```python
from build123d import *

# Parameters (mm, degrees)
F0_R     = 16.327253737
F0_R_2   = 12.7
F1_DEPTH = 101.6
F2_R     = 16.327253737
F3_DEPTH = 38.1
F3_TAPER = 22
F4_W     = 6.20650989
F4_H     = 11.6034736857
F5_DEPTH = 25.4
F7_DEPTH = 12.7
F8_COUNT = 3
F8_ANGLE = 240


with BuildPart() as f1:
    # F0 (on Front) → F1 (new body)
    with BuildSketch(Plane.XZ):
        Circle(F0_R)
        Circle(F0_R_2, mode=Mode.SUBTRACT)
    extrude(amount=F1_DEPTH)

    # F2 (on face) → F3 (join)
    with BuildSketch(Plane.XZ.offset(101.6)):
        Circle(F2_R)
    extrude(amount=F3_DEPTH, taper=F3_TAPER)

    # F4 (on Front) → F5 (join)
    with BuildSketch(Plane.XZ):
        with Locations((0.1349233789, 19.4290732034)):
            Rectangle(F4_W, F4_H)
    extrude(amount=F5_DEPTH)

    # F6 (on Right) → F7 (cut, symmetric)
    with BuildSketch(Plane.YZ):
        Polygon((25.9975232184, 33.8659547269), (-25.5434866995, 34.4056524336), (-25.8133374155, 16.5956672281), align=None)
    extrude(amount=F7_DEPTH, both=True, mode=Mode.SUBTRACT)

    # F8: F1 ×3 about axis
    f8_axis = Axis((0, 0, 0), (0, -1, 0))


with BuildPart() as f1_1:
    add(f1.part)
    for i in range(1, F8_COUNT):
        add(f1.part.rotate(f8_axis, i * F8_ANGLE / (F8_COUNT - 1)))


solid = f1_1.part
```
Could you check a few things on this model? Use its own coordinates, in mm. A direction names the side the tool comes from. Give positions to 0.01 mm unless a question says otherwise; leave off trailing zeros. Write each loop counter-clockwise with the first axis right and the second up, starting at its lowest first coordinate (ties: lowest second). Pieces come first, ordered by that corner, then holes. Notation, with made-up numbers: (6.25, 84) -> (42.25, 84) arc R8 ccw to (42.25, 98) -> close; hole circle Ø8 at (10.5, 20.5). An arc over 180 degrees is marked (long way). Write each question's results on one line, items separated by ' | '.
1. I want a section at D-D, the plane y = -129.5. Write out the boundary of the cut face in (x, z).
Check sheet entries:
outline: circle Ø10.11 at (0, 0)
2. On a 3-axis mill with a long thin cutter (end or side, diameter ignored), from which of +Z, -Z, +X, -X, +Y, -Y can I reach the whole of each face in a straight line? I mean faces 4 (the flat face through (18.41, -9.7, -7.2)), 5 (the flat face through (3.238, -10, 20)), 6 (the flat face through (0, -101.6, 0)), 7 (the flat face through (15.28, -9.7, -12.56)). Say none if no direction works.
Check sheet entries:
face 4: +X, +Y, -Y | face 5: +Z, +X, +Y, -Y | face 6: +Y | face 7: -Z, +Y, -Y
3. I need wall thicknesses on L1, parallel to Z at x = -0.5, y = -25.5; L2, parallel to X at y = -101, z = 11.5; L3, parallel to Z at x = -6, y = -9.5. Which ranges of each line are inside material? Lowest first, please.
Check sheet entries:
L1: z = -16.32 to -12.69, 12.69 to 16.32 | L2: x = -11.59 to -5.39, 5.39 to 11.59 | L3: z = -15.18 to -11.19, 11.19 to 15.18
4. Will these pins go through, and if not, where does the flat tip stop? pin 1 Ø4 at (x, y) = (16, -95.5) entering from -Z; pin 2 Ø1 at (x, z) = (3, -8) entering from -Y; pin 3 Ø23 at (x, z) = (0, 0) entering from +Y.
Check sheet entries:
pin 1: stops at z = -8.4 | pin 2: stops at y = -122.1 | pin 3: stops at y = -101.6
5. If we mould it in two halves opening along X, with no side actions, what happens to faces 1 (the cylindrical face through (-2.75, -50.09, -12.4)), 2 (the flat face through (7, 0, -11)), 3 (the flat face through (-2.968, -10, 20))? For each: released by +X, released by -X, zero draft, split by the parting line, or undercut.
Check sheet entries:
face 1: undercut | face 2: zero draft | face 3: released by -X
6. I want a section at A-A, the plane y = -22.5. Write out the boundary of the cut face in (x, z).
Check sheet entries:
outline: (-16.95, -6.05) -> (-13.84, -11.42) -> (-12.42, -10.6) arc R16.33 ccw to (12.24, -10.81) -> (13.71, -11.65) -> (16.81, -6.28) -> (15.39, -5.46) arc R16.33 ccw to (3.24, 16) -> (3.24, 17.7) -> (-2.97, 17.7) -> (-2.97, 16.06) arc R16.33 ccw to (-15.48, -5.2) -> close; hole circle Ø25.4 at (0, 0)
7. I want a section at B-B, the plane z = 22. Write out the boundary of the cut face in (x, y), then the cut area to 3 significant figures.
Check sheet entries:
outline: (-2.97, -9.6) -> (3.24, -9.6) -> (3.24, 0) -> (-2.97, 0) -> close | area: 59.6 mm²
8. I want a section at C-C, the plane y = -43. Write out the boundary of the cut face in (x, z).
Check sheet entries:
outline: circle Ø32.65 at (0, 0); hole circle Ø25.4 at (0, 0)
